Part model, mm, in its own coordinate system. A direction names the side the tool comes from. Give positions to 0.01 mm unless a question says otherwise; leave off trailing zeros. Order: outer loops, then holes, each group sorted by start corner. A loop starts at its lowest first (then second) coordinate and runs counter-clockwise, first axis right, second up.
1. Which spindle directions (+Z, -Z, +X, -X, +Y, -Y) get a long thin tool onto all of the face, cutting with end or side? Do faces 1 (the flat face through (-21.911, -26.553, 0.089)), 2 (the flat face through (11, -11, -6.35)). Say none if no direction does.
2. Probe line 1 (Y direction, x = -22, z = 2); line 2 (Y direction, x = -8, z = 2.25); line 3 (X direction, y = 7, z = 0). List the from-to ranges inside material, lowest first.
3. Drop flat-ended pins along their axis: pin 1 Ø2 at (x, z) = (-25.5, 4.5) entering from +Y; pin 2 Ø2 at (y, z) = (-37.5, -0.5) entering from -X; pin 3 Ø2 at (y, z) = (-39.5, -3) entering from -X. Give the stop position or say it passes through.
4. Slice it at C-C on z = 2. List the corners of the cut face in (x, y), and give its area (3 significant figures).
5. Slice it at B-B on x = -14. List the corners of the cut face in (y, z).
6. Slice it at D-D on y = 31.5. List the corners of the cut face in (x, z), and give its area (3 significant figures).
7. Mould opens along Y. For faces 3 (the flat face through (11, -11, 6.35)), 4 (the flat face through (25.72, -4, 0)), 5 (the cylindrical face through (-11.012, -49.592, 0.089)), 6 (the flat face through (-14.959, -28.734, 0.089)) say: +Y half, -Y half, draft (parallel to the pull), parting line (faces both ways), or undercut.
8. Slice it at A-A on x = 0. List the corners of the cut face in (y, z), and give its area (3 significant figures).
from build123d import *

# Parameters (mm, degrees)
F0_R     = 50.8
F0_R_2   = 12.7
F0_W     = 10.838795
F0_H     = 7.882758
F0_R_3   = 4.867285
F1_DEPTH = 6.35


with BuildPart() as f1:
    # F0 (on Top) → F1 (new body, symmetric)
    with BuildSketch(Plane.XY):
        Circle(F0_R)
        Polygon((-19.301308, -15.575219), (-10.737533, -18.357759), (-10.737533, -27.362245), (-19.301308, -30.144784), (-24.594012, -22.860002), align=None, mode=Mode.SUBTRACT)
        Circle(F0_R_2, mode=Mode.SUBTRACT)
        with Locations((31.139625, -3.941379)):
            Rectangle(F0_W, F0_H, mode=Mode.SUBTRACT)
        Polygon((-29.459082, 27.195517), (-5.329002, 27.726336), (-16.934339, 6.563665), align=None, mode=Mode.SUBTRACT)
        with Locations((24.079654, 19.813703)):
            Circle(F0_R_3, mode=Mode.SUBTRACT)
    extrude(amount=F1_DEPTH, both=True)


solid = f1.part
Data:
1. face 1: +Z, -Z
1. face 2: -Z, +X, -X, +Y, -Y
2. line 1: y = -45.79 to -26.43, -19.29 to 14.91, 27.36 to 45.79
2. line 2: y = -50.17 to -9.86, 9.86 to 22.86, 27.67 to 50.17
2. line 3: x = -50.32 to -17.2, -16.7 to -10.6, 10.6 to 50.32
3. pin 1: stops at y = 44.5
3. pin 2: stops at x = -35.33
3. pin 3: stops at x = -33.14
4. outline: circle Ø101.6 at (0, 0); hole (-29.46, 27.2) - (-16.93, 6.56) - (-5.33, 27.73) - close; hole (-24.59, -22.86) - (-19.3, -30.14) - (-10.74, -27.36) - (-10.74, -18.36) - (-19.3, -15.58) - close; hole circle Ø25.4 at (0, 0); hole circle Ø9.73 at (24.08, 19.81); hole (25.72, -7.88) - (36.56, -7.88) - (36.56, 0) - (25.72, 0) - close
4. area: 7,050 mm2
5. outline: (-48.83, -6.35) - (-28.42, -6.35) - (-28.42, 6.35) - (-48.83, 6.35) - close; (-17.3, -6.35) - (11.91, -6.35) - (11.91, 6.35) - (-17.3, 6.35) - close; (27.54, -6.35) - (48.83, -6.35) - (48.83, 6.35) - (27.54, 6.35) - close
6. outline: (-39.85, -6.35) - (39.85, -6.35) - (39.85, 6.35) - (-39.85, 6.35) - close
6. area: 1,010 mm2
7. face 3: draft
7. face 4: undercut
7. face 5: parting line
7. face 6: undercut
8. outline: (-50.8, -6.35) - (-12.7, -6.35) - (-12.7, 6.35) - (-50.8, 6.35) - close; (12.7, -6.35) - (50.8, -6.35) - (50.8, 6.35) - (12.7, 6.35) - close
8. area: 968 mm2
